```python
from build123d import *

# Parameters (mm, degrees)
SKETCH_3_R          = 1.6
SKETCH_3_R_2        = 6.75
SKETCH_3_R_3        = 2.1
EXTRUDE_1_DEPTH     = 5
FILLET_1_R          = 5
FILLET_2_R          = 1
SKETCH_4_R          = 3
CUT_EXTRUDE_1_DEPTH = 2
SKETCH_5_R          = 9.5
CUT_EXTRUDE_2_DEPTH = 2


with BuildPart() as part:
    # Sketch 3 → Extrude 1 (new body)
    with BuildSketch(Plane.XY):
        with BuildLine():
            Line((-1.982924342, 81.089990311), (28.095252633, 94.084080766))
            ThreePointArc((28.095252633, 94.084080766), (39.005008844, 94.166421351), (46.661147856, 86.393835167))
            Line((46.661147856, 86.393835167), (58.741421284, 55.937142786))
            ThreePointArc((58.741421284, 55.937142786), (59.091513319, 53.946870364), (58.625207696, 51.980577452))
            Line((58.625207696, 51.980577452), (53.071542706, 40.070704446))
            ThreePointArc((53.071542706, 40.070704446), (51.29898623, 42.316238157), (49.431489328, 44.483456058))
            ThreePointArc((49.431489328, 44.483456058), (49.497474683, 49.497474683), (44.483456058, 49.431489328))
            ThreePointArc((44.483456058, 49.431489328), (25.448448252, 61.437988912), (3.498787879, 66.407894737))
            ThreePointArc((3.498787879, 66.407894737), (0, 70), (-3.498787879, 66.407894737))
            ThreePointArc((-3.498787879, 66.407894737), (-6.351762076, 66.195959986), (-9.192980894, 65.861514576))
            Line((-9.192980894, 65.861514576), (-4.698463104, 78.210100717))
            ThreePointArc((-4.698463104, 78.210100717), (-3.637811921, 79.930207637), (-1.982924342, 81.089990311))
        make_face()
        with Locations((37.282933398, 90.008963455)):
            Circle(SKETCH_3_R, mode=Mode.SUBTRACT)
        with Locations((39.430674366, 73.695251163)):
            Circle(SKETCH_3_R, mode=Mode.SUBTRACT)
        with Locations((24.228714608, 79.99210907)):
            Circle(SKETCH_3_R, mode=Mode.SUBTRACT)
        with Locations((33.647440791, 81.232107896)):
            Circle(SKETCH_3_R_2, mode=Mode.SUBTRACT)
        with Locations((0, 76.5)):
            Circle(SKETCH_3_R_3, mode=Mode.SUBTRACT)
        with Locations((54.093668761, 54.093668761)):
            Circle(SKETCH_3_R_3, mode=Mode.SUBTRACT)
    extrude(amount=EXTRUDE_1_DEPTH)

    # Fillet 1
    fillet_1_edges = [part.edges().sort_by_distance(p)[0] for p in [
        (49.431489328, 44.483456058, 2.5),
        (44.483456058, 49.431489328, 2.5),
        (3.498787879, 66.407894737, 2.5),
        (-3.498787879, 66.407894737, 2.5),
    ]]
    fillet(fillet_1_edges, radius=FILLET_1_R)

    # Fillet 2
    fillet_2_edges = [part.edges().sort_by_distance(p)[0] for p in [
        (53.071542706, 40.070704446, 2.5),
        (-9.192980894, 65.861514576, 2.5),
    ]]
    fillet(fillet_2_edges, radius=FILLET_2_R)

    # Sketch 4 → Cut-Extrude 1 (cut)
    with BuildSketch(Plane.XY.offset(5)):
        with Locations((37.282933398, 90.008963455)):
            Circle(SKETCH_4_R)
        with Locations((39.430674366, 73.695251163)):
            Circle(SKETCH_4_R)
        with Locations((24.228714608, 79.99210907)):
            Circle(SKETCH_4_R)
    extrude(amount=-CUT_EXTRUDE_1_DEPTH, mode=Mode.SUBTRACT)

    # Sketch 5 → Cut-Extrude 2 (cut)
    with BuildSketch(Plane.XY.offset(5)):
        with Locations((33.647440791, 81.232107896)):
            Circle(SKETCH_5_R)
    extrude(amount=-CUT_EXTRUDE_2_DEPTH, mode=Mode.SUBTRACT)


solid = part.part
```
Here's how the part is built. I have some questions about the finished solid (model axes, mm). A direction names the side the tool comes from. Coordinates: 2 decimals unless noted, no trailing zeros. Order: outer loops, then holes, each group sorted by start corner. A loop starts at its lowest first (then second) coordinate and runs counter-clockwise, first axis right, second up.
Item 1: Thinking about a two-plate mould opening in X: for faces 3 (the face through (40.291, 75.044, 1.479)), 4 (the face through (38.86, 94.226, 2.465)), 5 (the face through (56.23, 46.84, 2.46)), which applies, pulls with the +X half, pulls with the -X half, needs draft (parallel to the pull), parting line crosses it, or undercut?
Response values:
face 3: undercut
face 4: parting line crosses it
face 5: pulls with the +X half
Item 2: I need wall thicknesses on probe 1 along X at (y, z) = (78, 4.7); probe 2 along X at (y, z) = (80.5, 3.45); probe 3 along Y at (x, z) = (38, 3.3). Which ranges of each line are inside material? Lowest first, please.
Response values:
probe 1: x = -4.77 to -1.47, 1.47 to 21.99, 42.58 to 49.99
probe 2: x = -3 to 21.27, 43.12 to 49
probe 3: y = 54.57 to 71.06, 92.92 to 94.54
Item 3: If we section it at A-A, the plane x = 33: List the corners of the cut face in (y, z) for me.
Response values:
outline: (57.73, 0) - (74.51, 0) - (74.51, 3) - (71.75, 3) - (71.75, 5) - (57.73, 5) - close; (87.95, 0) - (95.22, 0) - (95.22, 5) - (90.71, 5) - (90.71, 3) - (87.95, 3) - close
Item 4: Which directions (+Z, -Z, +X, -X, +Y, -Y) give clear straight access to the entire face, cutting with the end or side of a thin tool? Please do faces 1 (the face through (55.223, 55.864, 2.465)), 2 (the face through (38.5, 92.75, 4.01)).
Response values:
face 1: +Z, -Z
face 2: +Z
Item 5: I'm going to push flat-ended pins straight in: pin 1 Ø1 at (y, z) = (87, 4) entering from +X; pin 2 Ø3.5 at (x, y) = (54.09, 54.09) entering from +Z; pin 3 Ø3 at (x, z) = (29.5, 4) entering from -Y; pin 4 Ø5.5 at (x, y) = (37.28, 90.01) entering from +Z. Where does each tip first touch, or does it pass through?
Response values:
pin 1: stops at x = 46.62
pin 2: passes through
pin 3: stops at y = 58.83
pin 4: stops at z = 3
Item 6: If we section it at D-D, the plane y = 49: List the corners of the cut face in (x, z) for me.
Response values:
outline: (49.91, 0) - (57.24, 0) - (57.24, 5) - (49.91, 5) - close
Item 7: If we section it at B-B, the plane z = 4.3: Give the number of separate pieces and of enclosed holes in the cut face, then the cut area to 3 significant figures.
Response values:
separate pieces: 1
enclosed holes: 3
area: 1,390 mm2
Item 8: If we section it at C-C, the plane x = 0: List the corners of the cut face in (y, z) for me, then the cut area to 3 significant figures.
Response values:
outline: (70, 0) - (74.4, 0) - (74.4, 5) - (70, 5) - close; (78.6, 0) - (81.95, 0) - (81.95, 5) - (78.6, 5) - close
area: 38.7 mm2
